Job drawing, mm, ordinate dimensions from the low corner. One solid piece. A direction names the side the tool comes from. Coordinates: 2 decimals unless noted, no trailing zeros. Order: outer loops, then holes, each group sorted by start corner. A loop starts at its lowest first (then second) coordinate and runs counter-clockwise, first axis right, second up. Notation, with made-up numbers: (-13, -39.75) - (25, -39.75) arc R28 cw to (25, -0.75) - close; hole circle Ø2 at (22, 9). An arc over 180 degrees is marked (long way). Use one line per item in the form item = value.
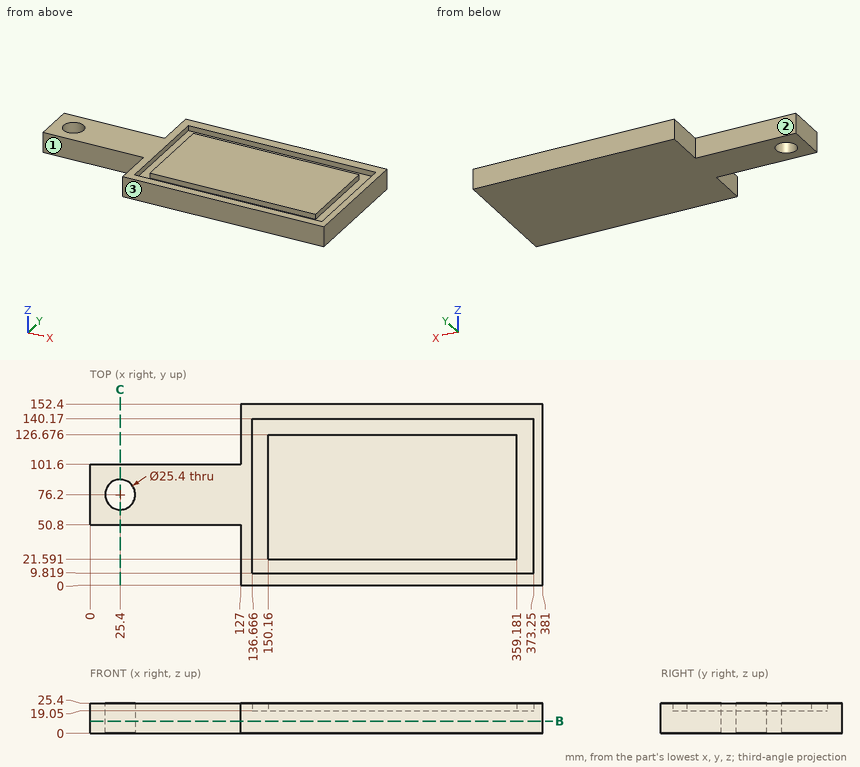
Item 1: Drill centre lines: line 1 (Y direction, x = 260, z = 23.75) (1 decimal); line 2 (Y direction, x = 25.4, z = 9.5); line 3 (X direction, y = 144, z = 21.5). Where is each one in solid material? Low to high. Write a range as [from, to].
Derived:
line_1 = [0, 9.8], [21.6, 126.7], [140.2, 152.4]
line_2 = [50.8, 63.5], [88.9, 101.6]
line_3 = [127, 381]
Item 2: 3-axis set-ups, long thin cutter, end or side, ignore diameter. For the marked faces 1, 2 and 3: which of +Z, -Z, +X, -X, +Y, -Y reach the whole face in a straight line?
Derived:
face_1 = +Z, -Z, -X, -Y
face_2 = +Z, -Z, -X, +Y
face_3 = +Z, -Z, +X, -X, -Y
Item 3: Drop flat-ended pins along their axis: pin 1 (5 mm diameter, centred on x = 306, z = 21, fed in from -Y); pin 2 (1.9 mm diameter, centred on y = 106.5, z = 23, fed in from -X); pin 3 (12 mm diameter, centred on x = 68, z = 16, fed in from +Y). Give the stop position or say it passes through.
Derived:
pin_1 = 0
pin_2 = 127
pin_3 = 101.6
Item 4: Cut at B-B, the plane z = 10.25. Write the cut outline in (x, y).
Derived:
outline = (0, 50.8) - (127, 50.8) - (127, 0) - (381, 0) - (381, 152.4) - (127, 152.4) - (127, 101.6) - (0, 101.6) - close; hole circle Ø25.4 at (25.4, 76.2)
Item 5: Cut at C-C, the plane x = 25.4. Write the cut outline in (y, z), plus the area to 3 significant figures.
Derived:
outline = (50.8, 0) - (63.5, 0) - (63.5, 25.4) - (50.8, 25.4) - close; (88.9, 0) - (101.6, 0) - (101.6, 25.4) - (88.9, 25.4) - close
area = 645 mm²
